from build123d import *

# Parameters (mm, degrees)
ESKIZ_KONTUR_R        = 30
PLASTINA_DEPTH        = 5
OTVERSTIYA_DEPTH      = 43.720018727
OTVERSTIYA_DEPTH_BACK = 43.720018727
ESKIZ_OTVERSTIYA_R    = 1.25
ESKIZ_OTVERSTIYA_R_2  = 23.75


with BuildPart() as part:
    # Eskiz_kontur → Plastina (new body)
    with BuildSketch(Plane.XY):
        Circle(ESKIZ_KONTUR_R)
    extrude(amount=PLASTINA_DEPTH)

    # Eskiz_otverstiya → Otverstiya (cut, two sides: drawn at the far end of the back side and taken through both)
    with BuildSketch(Plane.XY.offset(-OTVERSTIYA_DEPTH_BACK)):
        with Locations((0, -27)):
            Circle(ESKIZ_OTVERSTIYA_R)
        with Locations((-27, 0)):
            Circle(ESKIZ_OTVERSTIYA_R)
        Circle(ESKIZ_OTVERSTIYA_R_2)
        with Locations((27, 0)):
            Circle(ESKIZ_OTVERSTIYA_R)
        with Locations((0, 27)):
            Circle(ESKIZ_OTVERSTIYA_R)
    extrude(amount=OTVERSTIYA_DEPTH + OTVERSTIYA_DEPTH_BACK, mode=Mode.SUBTRACT)


solid = part.part
Could you check a few things on this model? Use its own coordinates, in mm. Coordinates: 2 decimals unless noted, no trailing zeros. Order: outer loops, then holes, each group sorted by start corner. A loop starts at its lowest first (then second) coordinate and runs counter-clockwise, first axis right, second up. Notation, with made-up numbers: (55, 30) - (91, 30) arc R13 cw to (91, 55) - close; hole circle Ø5 at (10, 4). An arc over 180 degrees is marked (long way). Answer in a Markdown table with one row per item. Add a question column.
(1) If we section it at D-D, the plane z = 2.5: Please give me the cut outline in (x, y), then the cut area to 3 significant figures.
(2) Will these pins go through, and if not, where does the flat tip stop? pin 1 (12 mm diameter, centred on x = -17.5, y = 0, fed in from +Z); pin 2 (2 mm diameter, centred on x = -19, z = 4.5, fed in from -Y).
(3) I need wall thicknesses on L1, parallel to Y at x = 0, z = 1.6; L2, parallel to Y at x = 10.5, z = 4.85; L3, parallel to X at y = 1, z = 1.3. Which ranges of each line are inside material? Lowest first, please.
(4) If we section it at A-A, the plane x = 0: Please give me the cut outline in (y, z).
(5) If we mould it in two halves opening along X, with no side actions, what happens to faces 1 (the face through (-29.97, 1.32, 2.46)), 2 (the face through (-0.27, -28.22, 2.46)), 3 (the face through (-0.27, 25.78, 2.46)), 4 (the face through (-22.4, -8.7, 0))? For each: released by +X, released by -X, zero draft, split by the parting line, or undercut.
(6) If we section it at B-B, the plane y = 22.5: Please give me the cut outline in (x, z).
Results are:
| question | item | result |
|---|---|---|
| 1 | outline | circle Ø60 at (0, 0); hole circle Ø2.5 at (-27, 0); hole circle Ø47.5 at (0, 0); hole circle Ø2.5 at (0, -27); hole circle Ø2.5 at (0, 27); hole circle Ø2.5 at (27, 0) |
| 1 | area | 1,040 mm2 |
| 2 | pin 1 | passes through |
| 2 | pin 2 | stops at y = -24 |
| 3 | L1 | y = -30 to -28.25, -25.75 to -23.75, 23.75 to 25.75, 28.25 to 30 |
| 3 | L2 | y = -28.1 to -21.3, 21.3 to 28.1 |
| 3 | L3 | x = -29.98 to -27.75, -26.25 to -23.73, 23.73 to 26.25, 27.75 to 29.98 |
| 4 | outline | (-30, 0) - (-28.25, 0) - (-28.25, 5) - (-30, 5) - close; (-25.75, 0) - (-23.75, 0) - (-23.75, 5) - (-25.75, 5) - close; (23.75, 0) - (25.75, 0) - (25.75, 5) - (23.75, 5) - close; (28.25, 0) - (30, 0) - (30, 5) - (28.25, 5) - close |
| 5 | face 1 | split by the parting line |
| 5 | face 2 | undercut |
| 5 | face 3 | undercut |
| 5 | face 4 | zero draft |
| 6 | outline | (-19.84, 0) - (-7.6, 0) - (-7.6, 5) - (-19.84, 5) - close; (7.6, 0) - (19.84, 0) - (19.84, 5) - (7.6, 5) - close |
